Check sheet for the modelled part. Datum: model origin and axes. Units: mm. A direction names the side the tool comes from. Give positions to 0.01 mm unless a question says otherwise; leave off trailing zeros. Order: outer loops, then holes, each group sorted by start corner. A loop starts at its lowest first (then second) coordinate and runs counter-clockwise, first axis right, second up. Notation, with made-up numbers: M 70.25,-1 L 110.25,-1 A25 cw 110.25,13 Z; hole C 34.5,-31 d8. An arc over 180 degrees is marked long. Return JSON: item names as keys, results as strings. Group by question number.
from build123d import *

# Parameters (mm, degrees)
SKETCH1_R            = 30
BASE_FLANGE1_DEPTH   = 1
EDGE_FLANGE1_START   = -75
EDGE_FLANGE1_DEPTH   = 140.5
EDGE_FLANGE1_START_2 = 65
EDGE_FLANGE1_2_DEPTH = 0.5
EDGE_FLANGE1_3_DEPTH = 140
SKETCH12_R           = 30
CUT_EXTRUDE1_DEPTH   = 10
EDGE_FLANGE2_START   = -65.5
EDGE_FLANGE2_DEPTH   = 131
EDGE_FLANGE2_2_DEPTH = 0.5
EDGE_FLANGE2_START_2 = 65
EDGE_FLANGE2_3_DEPTH = 0.5
EDGE_FLANGE2_START_3 = -65
EDGE_FLANGE2_4_DEPTH = 130
SKETCH16_R           = 30
CUT_EXTRUDE2_DEPTH   = 10
CUT_EXTRUDE3_DEPTH   = 10
FILLET2_R            = 9


# Read off the part's stored shape, not the designer's step: Edge-Flange1, Edge-Flange2
# Sheet-metal steps are written as plain solids
with BuildPart() as part:
    # Sketch1 → Base-Flange1 (new body)
    with BuildSketch(Plane(origin=(0, 0, 0), x_dir=(1, 0, 0), z_dir=(0, 1, 0))):
        with BuildLine():
            Line((-75, -65), (-75, 75))
            Line((-75, 75), (75, 75))
            Line((75, 75), (75, -65))
            ThreePointArc((75, -65), (72.071067812, -72.071067812), (65, -75))
            Line((65, -75), (-65, -75))
            ThreePointArc((-65, -75), (-72.071067812, -72.071067812), (-75, -65))
        make_face()
        with Locations(Location((0, 0, 0), (0, 0, 270))):
            Circle(SKETCH1_R, mode=Mode.SUBTRACT)
    extrude(amount=-BASE_FLANGE1_DEPTH)

    # Edge-Flange1 outline → Edge-Flange1 (cut)
    with BuildSketch(Plane.XY.offset(EDGE_FLANGE1_START)):
        with BuildLine():
            Line((-75, -1), (-73.279268401, -1))
            ThreePointArc((-73.279268401, -1), (-73.945137574, -0.867550387), (-74.509634201, -0.490365799))
            Line((-74.509634201, -0.490365799), (-75, 0))
            Line((-75, 0), (-75, -1))
        make_face()
        with BuildLine():
            ThreePointArc((74.509634201, -0.490365799), (73.945137574, -0.867550387), (73.279268401, -1))
            Line((73.279268401, -1), (75, -1))
            Line((75, -1), (75, 0))
            Line((75, 0), (74.509634201, -0.490365799))
        make_face()
    extrude(amount=EDGE_FLANGE1_DEPTH, mode=Mode.SUBTRACT)

    # Edge-Flange1 2 outline → Edge-Flange1 2 (cut)
    with BuildSketch(Plane.XY.offset(EDGE_FLANGE1_START_2)):
        with BuildLine():
            Line((-72.779268401, -1), (-72.779268401, 0))
            Line((-72.779268401, 0), (-75, 0))
            Line((-75, 0), (-74.509634201, -0.490365799))
            ThreePointArc((-74.509634201, -0.490365799), (-73.945137574, -0.867550387), (-73.279268401, -1))
            Line((-73.279268401, -1), (-72.779268401, -1))
        make_face()
        with BuildLine():
            Line((75, 0), (72.779268401, 0))
            Line((72.779268401, 0), (72.779268401, -1))
            Line((72.779268401, -1), (73.279268401, -1))
            ThreePointArc((73.279268401, -1), (73.945137574, -0.867550387), (74.509634201, -0.490365799))
            Line((74.509634201, -0.490365799), (75, 0))
        make_face()
    extrude(amount=EDGE_FLANGE1_2_DEPTH, mode=Mode.SUBTRACT)

    # Edge-Flange1 3 outline → Edge-Flange1 3 (add)
    with BuildSketch(Plane.XY.offset(EDGE_FLANGE1_START)):
        with BuildLine():
            Line((-75, 0), (-73.279268401, 0))
            ThreePointArc((-73.279268401, 0), (-73.562454141, 0.056329146), (-73.80252742, 0.216740982))
            Line((-73.80252742, 0.216740982), (-179.358910397, 105.773123959))
            Line((-179.358910397, 105.773123959), (-180.066017178, 105.066017178))
            Line((-180.066017178, 105.066017178), (-75, 0))
        make_face()
        with BuildLine():
            ThreePointArc((73.80252742, 0.216740982), (73.562454141, 0.056329146), (73.279268401, 0))
            Line((73.279268401, 0), (75, 0))
            Line((75, 0), (180.066017178, 105.066017178))
            Line((180.066017178, 105.066017178), (179.358910397, 105.773123959))
            Line((179.358910397, 105.773123959), (73.80252742, 0.216740982))
        make_face()
    extrude(amount=EDGE_FLANGE1_3_DEPTH)

    # Sketch12 → Cut-Extrude1 (cut)
    with BuildSketch(Plane(origin=(-36.792893219, -36.792893219, 0), x_dir=(0, 0, -1), z_dir=(0.7071067811865438, 0.7071067811865512, 0))):
        with Locations(Location((0, 126.618795027, 0), (0, 0, 90))):
            Circle(SKETCH12_R)
    cut_extrude1 = extrude(amount=-CUT_EXTRUDE1_DEPTH, mode=Mode.SUBTRACT)

    # Mirror1: Cut-Extrude1 across plane
    add(cut_extrude1.mirror(Plane(origin=(0, 0, 0), x_dir=(0, 0, 1), z_dir=(1, 0, 0))), mode=Mode.SUBTRACT)

    # Edge-Flange2 outline → Edge-Flange2 (cut)
    with BuildSketch(Plane.YZ.offset(EDGE_FLANGE2_START)):
        with BuildLine():
            ThreePointArc((-0.509634201, 74.509634201), (-0.132449613, 73.945137574), (0, 73.279268401))
            Line((0, 73.279268401), (0, 75))
            Line((0, 75), (-1, 75))
            Line((-1, 75), (-0.509634201, 74.509634201))
        make_face()
    extrude(amount=EDGE_FLANGE2_DEPTH, mode=Mode.SUBTRACT)

    # Edge-Flange2 2 outline → Edge-Flange2 2 (cut)
    with BuildSketch(Plane.YZ.offset(EDGE_FLANGE2_START)):
        with BuildLine():
            Line((-1, 72.779268401), (0, 72.779268401))
            Line((0, 72.779268401), (0, 73.279268401))
            ThreePointArc((0, 73.279268401), (-0.132449613, 73.945137574), (-0.509634201, 74.509634201))
            Line((-0.509634201, 74.509634201), (-1, 75))
            Line((-1, 75), (-1, 72.779268401))
        make_face()
    extrude(amount=EDGE_FLANGE2_2_DEPTH, mode=Mode.SUBTRACT)

    # Edge-Flange2 3 outline → Edge-Flange2 3 (cut)
    with BuildSketch(Plane.YZ.offset(EDGE_FLANGE2_START_2)):
        with BuildLine():
            Line((-1, 72.779268401), (0, 72.779268401))
            Line((0, 72.779268401), (0, 73.279268401))
            ThreePointArc((0, 73.279268401), (-0.132449613, 73.945137574), (-0.509634201, 74.509634201))
            Line((-0.509634201, 74.509634201), (-1, 75))
            Line((-1, 75), (-1, 72.779268401))
        make_face()
    extrude(amount=EDGE_FLANGE2_3_DEPTH, mode=Mode.SUBTRACT)

    # Edge-Flange2 4 outline → Edge-Flange2 4 (add)
    with BuildSketch(Plane.YZ.offset(EDGE_FLANGE2_START_3)):
        with BuildLine():
            ThreePointArc((-1.216740982, 73.80252742), (-1.056329146, 73.562454141), (-1, 73.279268401))
            Line((-1, 73.279268401), (-1, 75))
            Line((-1, 75), (-106.066017178, 180.066017178))
            Line((-106.066017178, 180.066017178), (-106.773123959, 179.358910397))
            Line((-106.773123959, 179.358910397), (-1.216740982, 73.80252742))
        make_face()
    extrude(amount=EDGE_FLANGE2_4_DEPTH)

    # Sketch16 → Cut-Extrude2 (cut)
    with BuildSketch(Plane(origin=(0, 37, 37), x_dir=(1, 0, 0), z_dir=(0, 0.7071067811865513, 0.7071067811865438))):
        with Locations(Location((0, -127.325901808, 0), (0, 0, 270))):
            Circle(SKETCH16_R)
    extrude(amount=-CUT_EXTRUDE2_DEPTH, mode=Mode.SUBTRACT)

    # Sketch17 → Cut-Extrude3 (cut)
    with BuildSketch(Plane(origin=(0, 0, 0), x_dir=(1, 0, 0), z_dir=(0, 1, 0))):
        Polygon((-72.779268401, -65), (-65, -65), (-65, -72.779268401), (-65.24665486, -73.060936269), (-65.339064279, -76.419683321), (-73.753182135, -79.834644684), (-76.575821569, -65.450165918), align=None)
    cut_extrude3 = extrude(amount=-CUT_EXTRUDE3_DEPTH, mode=Mode.SUBTRACT)

    # Mirror2: Cut-Extrude3 across plane
    add(cut_extrude3.mirror(Plane(origin=(0, 0, 0), x_dir=(0, 0, 1), z_dir=(1, 0, 0))), mode=Mode.SUBTRACT)

    # Fillet2
    fillet2_edges = [part.edges().sort_by_distance(p)[0] for p in [
        (-65, -0.5, 65),
    ]]
    fillet(fillet2_edges, radius=FILLET2_R)
    fillet2_2_edges = [part.edges().sort_by_distance(p)[0] for p in [
        (65, -0.5, 65),
    ]]
    fillet(fillet2_2_edges, radius=FILLET2_R)


solid = part.part
1) Release check for a two-part mould opening along X. For faces 4 (the face through (1.32, -0.49, -29.97)), 5 (the face through (-125.842, 52.256, -37.091)), 6 (the face through (67.566, -0.513, 67.706)), 7 (the face through (-0.91, -31.277, 103.863)) record: released by +X, released by -X, zero draft, split by the parting line, or undercut.
2) Sectioned sample at B-B on x = -58.5. Record the boundary of the cut face in (y, z), then the cut area to 3 significant figures.
3) Depth check by flat-ended pin: P1, Ø5, axis at x = -15.5, z = -47, coming from the -Y side; P2, Ø5, axis at x = -89, y = 21, coming from the +Z side. Enter the tip coordinate at first touch or a pass-through.
4) Sectioned sample at C-C on y = 23.5. Record the boundary of the cut face in (x, z).
5) Sectioned sample at A-A on z = -5. Record the boundary of the cut face in (x, y).
6) Material ranges on line 1 along X through (y, z) = (-0.5, 0); line 2 along X through (y, z) = (-0.8, 0); line 3 along Y through (x, z) = (-58.5, 2), recorded low to high.
7) Sectioned sample at D-D on x = 0. Record the boundary of the cut face in (y, z), then the cut area to 3 significant figures.
8) Tool access check on faces 1 (the face through (-105.48, 31.2, 1.32)), 2 (the face through (-32, -1, -2)), 3 (the face through (127.32, 53.734, -37.091)). Record the directions out of +Z, -Z, +X, -X, +Y, -Y that give a thin tool (end or side, any length) a straight path to the whole face; none if there is none.
Reply:
{
 "1": {"face 4": "undercut", "face 5": "undercut", "face 6": "released by +X", "face 7": "zero draft"},
 "2": {"outline": "M -106.77,179.36 L -1.22,73.8 A0.74 cw -1,73.28 L -1,-75 L 0,-75 L 0,73.28 A1.74 ccw -0.51,74.51 L -106.07,180.07 Z", "area": "299 mm^2"},
 "3": {"P1": "y = -1", "P2": "through"},
 "4": {"outline": "M -98.5,-75 L -97.09,-75 L -97.09,65 L -98.5,65 Z; M 97.09,-75 L 98.5,-75 L 98.5,65 L 97.09,65 Z"},
 "5": {"outline": "M -180.07,105.07 L -147.95,72.95 L -147.24,73.66 L -179.36,105.77 Z; M -106.12,31.12 L -74.51,-0.49 A1.74 ccw -73.28,-1 L -29.58,-1 L -29.58,0 L -73.28,0 A0.74 cw -73.8,0.22 L -105.41,31.82 Z; M 29.58,-1 L 73.28,-1 A1.74 ccw 74.51,-0.49 L 106.12,31.12 L 105.41,31.82 L 73.8,0.22 A0.74 cw 73.28,0 L 29.58,0 Z; M 147.24,73.66 L 147.95,72.95 L 180.07,105.07 L 179.36,105.77 Z"},
 "6": {"line 1": "-74.5 to -30, 30 to 74.5", "line 2": "-74.09 to -30, 30 to 74.09", "line 3": "-1 to 0"},
 "7": {"outline": "M -106.77,179.36 L -74.95,147.54 L -74.25,148.25 L -106.07,180.07 Z; M -32.53,105.11 L -1.22,73.8 A0.74 cw -1,73.28 L -1,30 L 0,30 L 0,73.28 A1.74 ccw -0.51,74.51 L -31.82,105.82 Z; M -1,-75 L 0,-75 L 0,-30 L -1,-30 Z", "area": "179 mm^2"},
 "8": {"face 1": "none", "face 2": "-Z, +X, -X, -Y", "face 3": "+Z, -Z, +Y"}
}
